```python
from build123d import *

# Parameters (mm, degrees)
CROQUIS1_R                = 6.35
CROQUIS1_R_2              = 6.26
CROQUIS1_R_3              = 6.25
SALIENTE_EXTRUIR1_DEPTH   = 7.9375
CROQUIS2_W                = 150
CROQUIS2_H                = 104.1375
SALIENTE_EXTRUIR2_DEPTH   = 7.9375
CONVERTIR_S_LIDO4_START   = -75
CONVERTIR_S_LIDO4_DEPTH   = 150
CONVERTIR_S_LIDO4_2_DEPTH = 150


# Read off the part's stored shape, not the designer's step: Convertir-Sólido4
with BuildPart() as part:
    # Croquis1 → Saliente-Extruir1 (new body)
    with BuildSketch(Plane.XY):
        with BuildLine():
            Line((-75, 16), (-75, 0))
            Line((-75, 0), (75, 0))
            Line((75, 0), (75, 54))
            ThreePointArc((75, 54), (60.355339059, 89.355339059), (25, 104))
            Line((25, 104), (-200, 104))
            ThreePointArc((-200, 104), (-235.355339059, 89.355339059), (-250, 54))
            Line((-250, 54), (-250, 0))
            ThreePointArc((-250, 0), (0, -250), (250, 0))
            ThreePointArc((250, 0), (200, 50), (150, 0))
            ThreePointArc((150, 0), (0, -150), (-150, 0))
            Line((-150, 0), (-150, 16))
            Line((-150, 16), (-75, 16))
        make_face()
        with BuildLine():
            ThreePointArc((-49.374105038, 47.65), (-55.724105038, 54), (-49.374105038, 60.35))
            Line((-49.374105038, 60.35), (49.374105038, 60.35))
            ThreePointArc((49.374105038, 60.35), (55.724105038, 54), (49.374105038, 47.65))
            Line((49.374105038, 47.65), (-49.374105038, 47.65))
        make_face(mode=Mode.SUBTRACT)
        with Locations((193.418858597, -50.883643138)):
            Circle(CROQUIS1_R, mode=Mode.SUBTRACT)
        with Locations((200, 0)):
            Circle(CROQUIS1_R_2, mode=Mode.SUBTRACT)
        with Locations((-100, -173.205080757)):
            Circle(CROQUIS1_R_3, mode=Mode.SUBTRACT)
        with Locations((-50.883643138, -193.418858597)):
            Circle(CROQUIS1_R, mode=Mode.SUBTRACT)
        with Locations((-140.775956893, -142.063823547)):
            Circle(CROQUIS1_R, mode=Mode.SUBTRACT)
        with Locations((-173.205080757, -100)):
            Circle(CROQUIS1_R, mode=Mode.SUBTRACT)
        with Locations((0, -200)):
            Circle(CROQUIS1_R_3, mode=Mode.SUBTRACT)
        with Locations((52.642901704, -192.947466685)):
            Circle(CROQUIS1_R, mode=Mode.SUBTRACT)
        with Locations((100, -173.205080757)):
            Circle(CROQUIS1_R_3, mode=Mode.SUBTRACT)
        with Locations((142.063823547, -140.775956893)):
            Circle(CROQUIS1_R, mode=Mode.SUBTRACT)
        with Locations((173.205080757, -100)):
            Circle(CROQUIS1_R_3, mode=Mode.SUBTRACT)
        with Locations((-192.947466685, -52.642901704)):
            Circle(CROQUIS1_R, mode=Mode.SUBTRACT)
        with Locations((-200, 0)):
            Circle(CROQUIS1_R, mode=Mode.SUBTRACT)
        with Locations((-200, 54)):
            Circle(CROQUIS1_R, mode=Mode.SUBTRACT)
    extrude(amount=SALIENTE_EXTRUIR1_DEPTH)

    # Croquis2 → Saliente-Extruir2 (add)
    with BuildSketch(Plane.XZ):
        with Locations((0, 52.06875)):
            Rectangle(CROQUIS2_W, CROQUIS2_H)
        with BuildLine():
            Line((-50.16849794, 72.5375), (50.16849794, 72.5375))
            ThreePointArc((50.16849794, 72.5375), (56.66849794, 66.0375), (50.16849794, 59.5375))
            Line((50.16849794, 59.5375), (-50.16849794, 59.5375))
            ThreePointArc((-50.16849794, 59.5375), (-56.66849794, 66.0375), (-50.16849794, 72.5375))
        make_face(mode=Mode.SUBTRACT)
    extrude(amount=-SALIENTE_EXTRUIR2_DEPTH)

    # Convertir-Sólido4 outline → Convertir-Sólido4 (cut)
    with BuildSketch(Plane.YZ.offset(CONVERTIR_S_LIDO4_START)):
        with BuildLine():
            Line((0, 12.9375), (0, 0))
            Line((0, 0), (12.9375, 0))
            ThreePointArc((12.9375, 0), (3.789306018, 3.789306018), (0, 12.9375))
        make_face()
    extrude(amount=CONVERTIR_S_LIDO4_DEPTH, mode=Mode.SUBTRACT)

    # Convertir-S_lido4 2 outline → Convertir-S_lido4 2 (add)
    with BuildSketch(Plane.YZ.offset(CONVERTIR_S_LIDO4_START)):
        with BuildLine():
            Line((7.9375, 12.9375), (7.9375, 7.9375))
            Line((7.9375, 7.9375), (12.9375, 7.9375))
            ThreePointArc((12.9375, 7.9375), (9.401966094, 9.401966094), (7.9375, 12.9375))
        make_face()
    extrude(amount=CONVERTIR_S_LIDO4_2_DEPTH)


solid = part.part
```
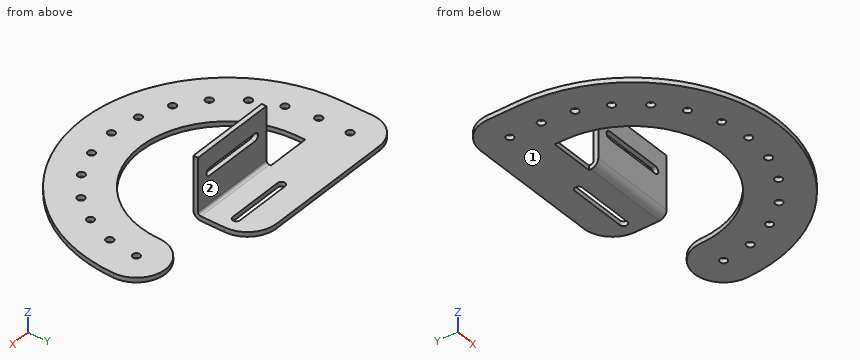
CAD build for the part. Positions are in the model's coordinates, mm. Face numbers are marked on the shaded views. A direction names the side the tool comes from. Give positions to 0.01 mm unless a question says otherwise; leave off trailing zeros. Write each loop counter-clockwise with the first axis right and the second up, starting at its lowest first coordinate (ties: lowest second). Pieces come first, ordered by that corner, then holes. Notation, with made-up numbers: (70.5, -7.75) -> (88.5, -7.75) arc R21 cw to (88.5, -1.75) -> close; hole circle Ø10 at (-10.5, 77.5). An arc over 180 degrees is marked (long way). Write each question's results on one line, items separated by ' | '.
1. Which spindle directions (+Z, -Z, +X, -X, +Y, -Y) get a long thin tool onto all of the face, cutting with end or side? Do the marked faces 1 and 2. Say none if no direction does.
Geometry check:
face 1: -Z, +X, -X, +Y, -Y | face 2: +Z, +X, -X, +Y
2. Cut at A-A, the plane x = 16. Give the number of separate pieces and of enclosed holes in the cut face, then the cut area to 3 significant figures.
Geometry check:
separate pieces: 4 | enclosed holes: 0 | area: 2,150 mm²
3. Wall check: probe 1 along Z at (x, y) = (-205, 11). Give the ranges that are in metal, low to high. Write a range as [from, to].
Geometry check:
probe 1: [0, 7.94]
4. Cut at C-C, the plane x = 100. Write the cut outline in (y, z), then the cut area to 3 significant figures.
Geometry check:
outline: (-229.13, 0) -> (-179.46, 0) -> (-179.46, 7.94) -> (-229.13, 7.94) -> close; (-166.96, 0) -> (-111.8, 0) -> (-111.8, 7.94) -> (-166.96, 7.94) -> close | area: 832 mm²
5. Drop flat-ended pins along their axis: P1, Ø10, axis at x = 100, y = -173.21, coming from the +Z side; P2, Ø16.5, axis at x = -200, y = 0, coming from the +Z side; P3, Ø8, axis at x = 72.5, z = 13, coming from the -Y side. Give the stop position or say it passes through.
Geometry check:
P1: through | P2: z = 7.94 | P3: y = 0
6. Cut at D-D, the plane z = 26. Write the cut outline in (x, y), then the cut area to 3 significant figures.
Geometry check:
outline: (-75, 0) -> (75, 0) -> (75, 7.94) -> (-75, 7.94) -> close | area: 1,190 mm²
7. Cut at B-B, the plane y = -66.5. Write the cut outline in (x, z).
Geometry check:
outline: (-240.99, 0) -> (-134.45, 0) -> (-134.45, 7.94) -> (-240.99, 7.94) -> close; (134.45, 0) -> (240.99, 0) -> (240.99, 7.94) -> (134.45, 7.94) -> close
